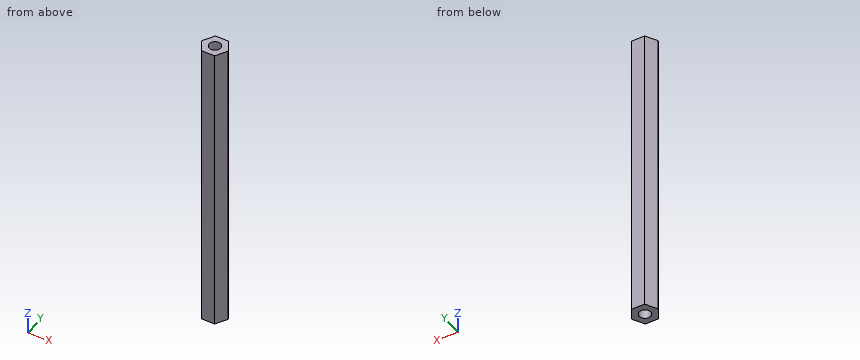
Autodesk Inventor part; units mm, degrees
ref_plane "Work Plane1" through (0, 0, 82.3722) normal (0, 0, -1) x (-1, 0, 0)
ref_plane "YZ Plane" through (0, 0, 0) normal (1, 0, 0) x (0, 1, 0)
ref_plane "XZ Plane" through (0, 0, 0) normal (0, 1, 0) x (-1, 0, 0)
sketch "Sketch1" plane through (0, 0, 0) normal (0, 0, 1) x (1, 0, 0)
  line L0 (-3.6662, 6.35) -> (3.6662, 6.35)
  line L1 (3.6662, 6.35) -> (7.3323, 0)
  line L2 (7.3323, 0) -> (3.6662, -6.35)
  line L3 (3.6662, -6.35) -> (-3.6662, -6.35)
  line L4 (-3.6662, -6.35) -> (-7.3323, 0)
  line L5 (-7.3323, 0) -> (-3.6662, 6.35)
  point P0 (0, 0)
  point P1 (0, 0)
  dimension "d0" = 12.7
extrude "Extrusion1" add sketch "Sketch1" along normal blind 164.7444
ref_plane "Work Plane1" through (0, 0, 82.3722) normal (0, 0, -1) x (-1, 0, 0)
sketch "Sketch2" plane through (0, 0, 164.7444) normal (0, 0, 1) x (1, 0, 0)
  point P0 (0, 0)
  point P1 (0, 0)
hole "Hole1" at (0, 0, 164.7444) direction (0, 0, -1) diameter 6.35 depth 38.1 tip angle 118
thread "Thread1"
mirror "Mirror1" about plane through (0, 0, 82.3722) normal (0, 0, -1) of "Hole1"
properties part number "Steel Shaft for Jeep" material "Steel, Carbon"
Work out the finished part from the listing and answer in its coordinate system (mm). Coordinates: 2 decimals unless noted, no trailing zeros. Write each loop counter-clockwise with the first axis right and the second up, starting at its lowest first coordinate (ties: lowest second). Pieces come first, ordered by that corner, then holes. Notation, with made-up numbers: (-16.75, -23) - (3.25, -23) arc R17 cw to (3.25, 5) - close; hole circle Ø4 at (-12, -28.75). An arc over 180 degrees is marked (long way). Answer as a JSON object with one key per item and string values.
Q1. Find section A-A (z = 15). Write down the section's boundary in (x, y) (3 decimals), plus the area to 3 significant figures.
Results list:
{"outline": "(-7.332, 0) - (-3.666, -6.35) - (3.666, -6.35) - (7.332, 0) - (3.666, 6.35) - (-3.666, 6.35) - close; hole circle Ø6.35 at (0, 0)", "area": "108 mm^2"}
Q2. Find section B-B (z = 103.5). Write down the section's boundary in (x, y).
Results list:
{"outline": "(-7.33, 0) - (-3.67, -6.35) - (3.67, -6.35) - (7.33, 0) - (3.67, 6.35) - (-3.67, 6.35) - close"}
Q3. Given pin 1 Ø1.5 at (x, y) = (-2.5, 1.5) entering from +Z; pin 2 Ø3 at (y, z) = (-3.5, 102) entering from -X; pin 3 Ø3 at (y, z) = (-1, 122.5) entering from -X; pin 4 Ø4 at (x, y) = (0, 0) entering from -Z, each flat-ended and moving along its own axis, determine where each tip first touches the part or whether it passes through.
Results list:
{"pin 1": "stops at z = 164.74", "pin 2": "stops at x = -6.18", "pin 3": "stops at x = -7.33", "pin 4": "stops at z = 38.81"}
Q4. Consider L1, parallel to Y at x = 0, z = 127.5 (3 decimals); L2, parallel to X at y = 0, z = 9.5 (3 decimals); L3, parallel to X at y = 1.5, z = 136. Determine where each line is inside the solid, lowest interval first. Write a range as from..to.
Results list:
{"L1": "y = -6.35..-3.175, 3.175..6.35", "L2": "x = -7.332..-3.175, 3.175..7.332", "L3": "x = -6.47..-2.8, 2.8..6.47"}
